from build123d import *

# Parameters (mm, degrees)
SKETCH2_R                  = 75.946
BOSS_EXTRUDE1_DEPTH        = 12.7
SKETCH3_R                  = 5.55625
CUT_EXTRUDE1_DEPTH         = 1
CUT_EXTRUDE1_DEPTH_BACK    = 13.7
CIRPATTERN2_COUNT          = 4
CIRPATTERN2_ANGLE          = 270
SKETCH11_R                 = 69.596
CUT_EXTRUDE2_DEPTH         = 6.35
F_10_24_TAPPED_HOLE1_D     = 3.7973
F_10_24_TAPPED_HOLE1_DEPTH = 12.82954
F_10_24_TAPPED_HOLE1_TIP   = 1.140824014


with BuildPart() as part:
    # Sketch2 → Boss-Extrude1 (new body)
    with BuildSketch(Plane(origin=(0, 0, 0), x_dir=(1, 0, 0), z_dir=(0, 1, 0))):
        Circle(SKETCH2_R)
    extrude(amount=BOSS_EXTRUDE1_DEPTH)

    # Sketch3 → Cut-Extrude1 (cut, two sides)
    with BuildSketch(Plane(origin=(0, 12.7, 0), x_dir=(1, 0, 0), z_dir=(0, 1, 0))) as cut_extrude1_sk:
        Circle(SKETCH3_R)
    extrude(amount=CUT_EXTRUDE1_DEPTH, mode=Mode.SUBTRACT)
    extrude(cut_extrude1_sk.sketch, amount=-CUT_EXTRUDE1_DEPTH_BACK, mode=Mode.SUBTRACT)

    # Sketch10 → 1/4-20 Tapped Hole1 (revolve, cut)
    with BuildSketch(Plane(origin=(-76.1746, 6.35, 0), x_dir=(0, 0, 1), z_dir=(0, 1, 0))):
        Polygon((0, 0), (0, 26.933816902), (2.5527, 25.4), (2.5527, 0), align=None)
    f_1_4_20_tapped_hole1 = revolve(axis=Axis((-82.5246, 6.35, 0), (1, 0, 0)), mode=Mode.SUBTRACT)

    # CirPattern2: 1/4-20 Tapped Hole1 ×4 about axis
    cirpattern2_axis = Axis((0, 12.7, 0), (0, -1, 0))
    for i in range(1, CIRPATTERN2_COUNT):
        add(f_1_4_20_tapped_hole1.rotate(cirpattern2_axis, i * CIRPATTERN2_ANGLE / (CIRPATTERN2_COUNT - 1)), mode=Mode.SUBTRACT)

    # Sketch11 → Cut-Extrude2 (cut)
    with BuildSketch(Plane.XZ):
        Circle(SKETCH11_R)
    extrude(amount=-CUT_EXTRUDE2_DEPTH, mode=Mode.SUBTRACT)

    # #10-24 Tapped Hole1
    with Locations(Plane(origin=(0, 12.7, 0), x_dir=(1, 0, 0), z_dir=(0, 1, 0))):
        with Locations((0, 0), (44.901280605, 44.901280605), (44.901280605, -44.901280605), (-44.901280605, -44.901280605), (-44.901280605, 44.901280605)):
            Hole(F_10_24_TAPPED_HOLE1_D / 2, depth=F_10_24_TAPPED_HOLE1_DEPTH)
            with Locations((0, 0, -(F_10_24_TAPPED_HOLE1_DEPTH + F_10_24_TAPPED_HOLE1_TIP / 2))):  # 118° drill point
                Cone(0, F_10_24_TAPPED_HOLE1_D / 2, F_10_24_TAPPED_HOLE1_TIP, mode=Mode.SUBTRACT)


solid = part.part
Source: CAD feature listing. Evaluate the final solid. Frame: model axes, mm. A direction names the side the tool comes from. Give positions to 0.01 mm unless a question says otherwise; leave off trailing zeros. Write each loop counter-clockwise with the first axis right and the second up, starting at its lowest first coordinate (ties: lowest second). Pieces come first, ordered by that corner, then holes. Notation, with made-up numbers: M -23,75 L 34,75 A25 ccw 34,95 Z; hole C -24.75,-40 d3. An arc over 180 degrees is marked long. Answer as a JSON object with one key per item and string values.
Q1. Access query for faces 1 (the face through (1.178, 8.615, 66.333)), 2 (the face through (-1.178, 8.615, -66.333)), 3 (the face through (-66.333, 8.615, 1.178)), 4 (the face through (-15.09, 3.13, -67.94)), 5 (the face through (66.333, 8.615, -1.178)). Directions: +Z, -Z, +X, -X, +Y, -Y. A direction counts if a zero-diameter tool reaches every point of the face in a straight line with its end or side. Return the directions, or none.
Geometry check:
{"face 1": "+Z", "face 2": "-Z", "face 3": "-X", "face 4": "-Y", "face 5": "+X"}
Q2. Cut plane B-B, the plane x = 0. Return the cut outline in (y, z), then the cut area to 3 significant figures.
Geometry check:
{"outline": "M 0,-75.95 L 3.8,-75.95 L 3.8,-69.6 L 0,-69.6 Z; M 0,69.6 L 3.8,69.6 L 3.8,75.95 L 0,75.95 Z; M 6.35,-49.24 L 8.9,-50.77 L 8.9,-75.95 L 12.7,-75.95 L 12.7,-5.56 L 6.35,-5.56 Z; M 6.35,5.56 L 12.7,5.56 L 12.7,75.95 L 8.9,75.95 L 8.9,50.77 L 6.35,49.24 Z", "area": "810 mm^2"}
Q3. Ray query, line 1 along Y through (x, z) = (7.5, -45); line 2 along X through (y, z) = (2.25, 46.5); line 3 along X through (y, z) = (7.75, 60). Return the intervals inside material, ascending.
Geometry check:
{"line 1": "y = 6.35 to 12.7", "line 2": "x = -60.05 to -51.78, 51.78 to 60.05", "line 3": "x = -46.56 to -2.13, 2.13 to 46.56"}
Q4. Mould query, pull axis X, two halves, no side actions, for faces 6 (the face through (5.3, 9.57, -1.67)), 7 (the face through (33, 0, 62)), 8 (the face through (72.44, 6.26, -22.81)). Classes: +X half, -X half, draft (parallel to the pull), parting line (faces both ways), or undercut.
Geometry check:
{"face 6": "undercut", "face 7": "draft", "face 8": "parting line"}
Q5. Cut plane C-C, the plane z = -57. Return the cut outline in (x, y), then the cut area to 3 significant figures.
Geometry check:
{"outline": "M -50.19,0 L -39.93,0 L -39.93,6.35 L -2.55,6.35 A2.55 cw 2.55,6.35 L 39.93,6.35 L 39.93,0 L 50.19,0 L 50.19,12.7 L -50.19,12.7 Z", "area": "757 mm^2"}
Q6. Contact query for flat-ended pins moving along their axis: P1, Ø2, axis at x = -15.5, y = 4.5, coming from the +Z side; P2, Ø3, axis at y = 6.35, z = 0, coming from the +X side; P3, Ø10, axis at x = 8, z = 34.5, coming from the -Y side. Output: stop coordinate, or through.
Geometry check:
{"P1": "stops at z = 74.55", "P2": "stops at x = 50.14", "P3": "stops at y = 6.35"}
Q7. Cut plane A-A, the plane z = 0. Return the cut outline in (x, y), then the cut area to 3 significant figures.
Geometry check:
{"outline": "M -75.95,0 L -69.6,0 L -69.6,3.8 L -75.95,3.8 Z; M -75.95,8.9 L -50.77,8.9 L -49.24,6.35 L -5.56,6.35 L -5.56,12.7 L -75.95,12.7 Z; M 5.56,6.35 L 49.24,6.35 L 50.77,8.9 L 75.95,8.9 L 75.95,12.7 L 5.56,12.7 Z; M 69.6,0 L 75.95,0 L 75.95,3.8 L 69.6,3.8 Z", "area": "810 mm^2"}
Q8. Cut plane D-D, the plane x = 60. Return the cut outline in (y, z).
Geometry check:
{"outline": "M 0,-46.56 L 12.7,-46.56 L 12.7,46.56 L 0,46.56 L 0,35.26 L 6.35,35.26 L 6.35,2.55 A2.55 cw 6.35,-2.55 L 6.35,-35.26 L 0,-35.26 Z"}
